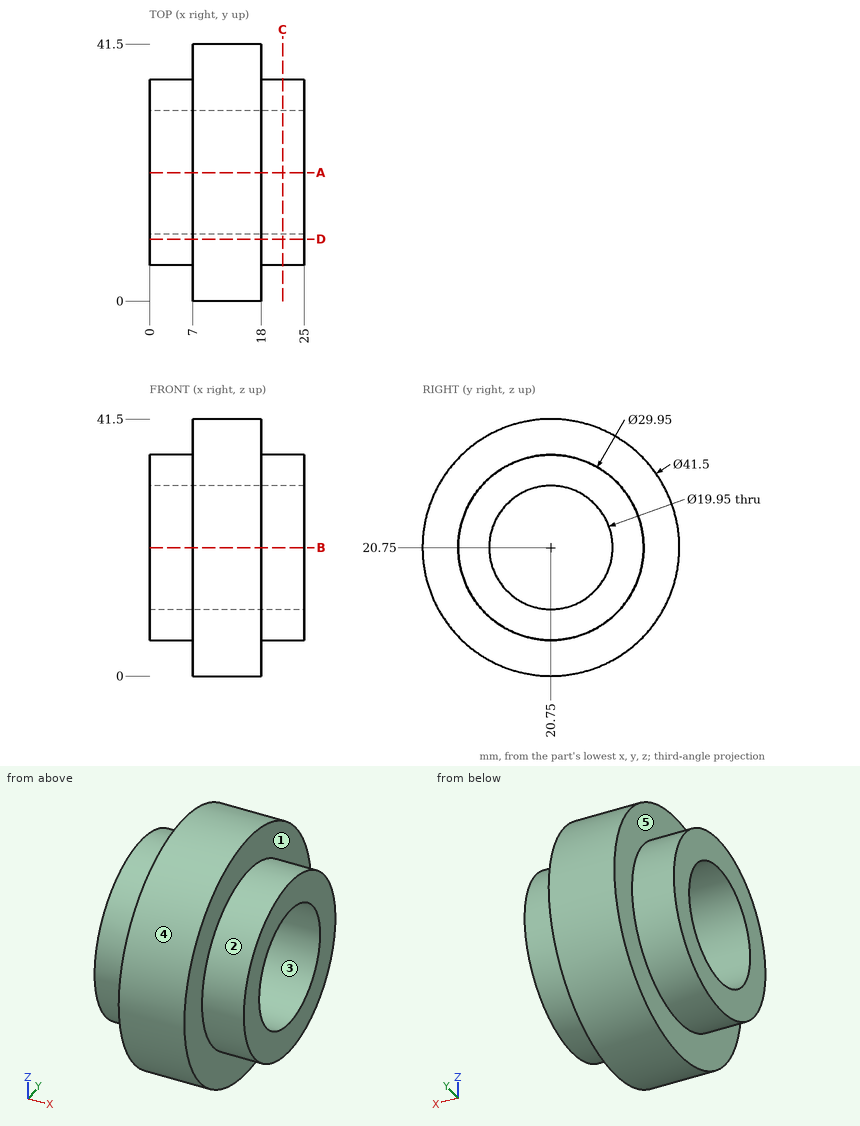
Drawing for the job (mm, zero at the part's lowest x, y, z). A direction names the side the tool comes from. Round coordinates to 2 decimals unless told otherwise and drop trailing zeros. Write each loop counter-clockwise with the first axis right and the second up, starting at its lowest first coordinate (ties: lowest second). Pieces come first, ordered by that corner, then holes. Notation, with made-up numbers: M 53,-26 L 85,-26 A13 cw 85,-9 Z; hole C -9,44.5 d3. An arc over 180 degrees is marked long. Answer as a JSON object with one key per item and string values. Group by question number.
(1) Mould opens along Z. For the marked faces 1, 2 and 3 say: pulls with the +Z half, pulls with the -Z half, needs draft (parallel to the pull), parting line crosses it, or undercut.
(2) Drill centre lines: L1, parallel to Y at x = 5.25, z = 20.75 (3 decimals); L2, parallel to Y at x = 8.75, z = 20.75 (3 decimals); L3, parallel to Z at x = 16, y = 21. Where is each one in solid material? Low to high.
(3) Cut at A-A (y = 20.75). Give the cut face in (x, z) (3 decimals), and give its area (3 significant figures).
(4) Which spindle directions (+Z, -Z, +X, -X, +Y, -Y) get a long thin tool onto all of the face, cutting with end or side? Do the marked faces 4 and 5. Say none if no direction does.
(5) Cut at D-D (y = 10). Give the cut face in (x, z), and give its area (3 significant figures).
(6) Flat gauge pins, fed straight in: pin 1 (10 mm diameter, centred on x = 17.5, z = 27, fed in from -Y); pin 2 (3 mm diameter, centred on x = 21, y = 16, fed in from +Z); pin 3 (3 mm diameter, centred on x = 21, z = 32.5, fed in from -Y). Where does each tip first touch, or does it go through?
(7) Cut at C-C (x = 21.5). Give the cut face in (y, z) (3 decimals), and give its area (3 significant figures).
Responses:
{
 "1": {"face 1": "needs draft", "face 2": "parting line crosses it", "face 3": "undercut"},
 "2": {"L1": "y = 5.775 to 10.775, 30.725 to 35.725", "L2": "y = 0 to 10.775, 30.725 to 41.5", "L3": "z = 0 to 10.78, 30.72 to 41.5"},
 "3": {"outline": "M 0,5.775 L 7,5.775 L 7,0 L 18,0 L 18,5.775 L 25,5.775 L 25,10.775 L 0,10.775 Z; M 0,30.725 L 25,30.725 L 25,35.725 L 18,35.725 L 18,41.5 L 7,41.5 L 7,35.725 L 0,35.725 Z", "area": "377 mm2"},
 "4": {"face 4": "+X, -X", "face 5": "-X"},
 "5": {"outline": "M 0,10.32 L 7,10.32 L 7,3 L 18,3 L 18,10.32 L 25,10.32 L 25,31.18 L 18,31.18 L 18,38.5 L 7,38.5 L 7,31.18 L 0,31.18 Z", "area": "682 mm2"},
 "6": {"pin 1": "stops at y = 0.04", "pin 2": "stops at z = 35.37", "pin 3": "stops at y = 9.83"},
 "7": {"outline": "C 20.75,20.75 d29.95; hole C 20.75,20.75 d19.95", "area": "392 mm2"}
}
